Geometry check sheet. Reference: the model listing, model coordinates, mm. A direction names the side the tool comes from. Give positions to 0.01 mm unless a question says otherwise; leave off trailing zeros. Order: outer loops, then holes, each group sorted by start corner. A loop starts at its lowest first (then second) coordinate and runs counter-clockwise, first axis right, second up.
from build123d import *

# Parameters (mm, degrees)
SKETCH1_W           = 146.05
SKETCH1_H           = 146.05
SKETCH1_R           = 3.175
BOSS_EXTRUDE1_DEPTH = 3.175
SKETCH4_W           = 12.7
SKETCH4_H           = 12.7
BOSS_EXTRUDE4_DEPTH = 9.525
SKETCH6_W           = 5.935
SKETCH6_H           = 6
CUT_EXTRUDE2_DEPTH  = 150
SKETCH7_W           = 5.935
SKETCH7_H           = 6
CUT_EXTRUDE3_DEPTH  = 15
SKETCH2_R           = 1.5
CUT_EXTRUDE4_DEPTH  = 15
FILLET2_R           = 3.175


with BuildPart() as part:
    # Sketch1 → Boss-Extrude1 (new body)
    with BuildSketch(Plane(origin=(0, 0, 0), x_dir=(1, 0, 0), z_dir=(0, 1, 0))):
        with Locations((73.025, 73.025)):
            Rectangle(SKETCH1_W, SKETCH1_H)
        with Locations(Location((133.35, 12.7, 0), (0, 0, 270))):
            Circle(SKETCH1_R, mode=Mode.SUBTRACT)
        with Locations(Location((82.55, 12.7, 0), (0, 0, 270))):
            Circle(SKETCH1_R, mode=Mode.SUBTRACT)
    extrude(amount=BOSS_EXTRUDE1_DEPTH)

    # Sketch4 → Boss-Extrude4 (add)
    with BuildSketch(Plane(origin=(0, 3.175, 0), x_dir=(1, 0, 0), z_dir=(0, 1, 0))):
        with Locations((10.648879027, 12.7)):
            Rectangle(SKETCH4_W, SKETCH4_H)
        with Locations((10.648879027, 125.73)):
            Rectangle(SKETCH4_W, SKETCH4_H)
        with Locations((133.838879027, 125.73)):
            Rectangle(SKETCH4_W, SKETCH4_H)
    extrude(amount=BOSS_EXTRUDE4_DEPTH)

    # Sketch6 → Cut-Extrude2 (cut)
    with BuildSketch(Plane.XY.offset(-6.35)):
        with Locations((10.648879027, 6.175)):
            Rectangle(SKETCH6_W, SKETCH6_H)
    extrude(amount=-CUT_EXTRUDE2_DEPTH, mode=Mode.SUBTRACT)

    # Sketch7 → Cut-Extrude3 (cut)
    with BuildSketch(Plane.XY.offset(-119.38)):
        with Locations((133.838879027, 6.175)):
            Rectangle(SKETCH7_W, SKETCH7_H)
    extrude(amount=-CUT_EXTRUDE3_DEPTH, mode=Mode.SUBTRACT)

    # Sketch2 → Cut-Extrude4 (cut)
    with BuildSketch(Plane(origin=(0, 3.175, 0), x_dir=(1, 0, 0), z_dir=(0, 1, 0))):
        with Locations(Location((10.648879027, 125.73, 0), (0, 0, 90))):
            Circle(SKETCH2_R)
        with Locations(Location((133.838879027, 125.73, 0), (0, 0, 180))):
            Circle(SKETCH2_R)
        with Locations(Location((10.648879027, 12.7, 0), (0, 0, 90))):
            Circle(SKETCH2_R)
    extrude(amount=CUT_EXTRUDE4_DEPTH, mode=Mode.SUBTRACT)

    # Fillet2
    # the kernel refuses this fillet: 3.175 mm, written as the material it adds along each edge
    with BuildSketch(Plane(origin=(136.806379027, 9.175, -119.38), x_dir=(0, -1, 0), z_dir=(0, 0, -1))) as fillet2_piece_1_section:
        with BuildLine():
            CenterArc((FILLET2_R, FILLET2_R), FILLET2_R, 180, 90)
            Line((0, FILLET2_R), (0, 0))
            Line((0, 0), (FILLET2_R, 0))
        make_face()
    fillet2_piece_1 = extrude(amount=12.7, mode=Mode.PRIVATE)
    fillet2_piece_1 = fillet2_piece_1 - Plane(origin=(133.838879027, 8.440537645, -125.73), x_dir=(-1, 0, 0), z_dir=(0, -1, 0)) * Cylinder(1.5, 39, mode=Mode.PRIVATE)
    add(fillet2_piece_1)
    with BuildSketch(Plane(origin=(130.871379027, 9.175, -119.38), x_dir=(0, -1, 0), z_dir=(0, 0, -1))) as fillet2_piece_2_section:
        with BuildLine():
            CenterArc((FILLET2_R, -FILLET2_R), FILLET2_R, 90, 90)
            Line((0, -FILLET2_R), (0, 0))
            Line((0, 0), (FILLET2_R, 0))
        make_face()
    fillet2_piece_2 = extrude(amount=12.7, mode=Mode.PRIVATE)
    fillet2_piece_2 = fillet2_piece_2 - Plane(origin=(133.838879027, 8.44053751, -125.73), x_dir=(-1, 0, 0), z_dir=(0, -1, 0)) * Cylinder(1.5, 39, mode=Mode.PRIVATE)
    add(fillet2_piece_2)
    with BuildSketch(Plane(origin=(13.616379027, 9.175, -119.38), x_dir=(0, -1, 0), z_dir=(0, 0, -1))) as fillet2_piece_3_section:
        with BuildLine():
            CenterArc((FILLET2_R, FILLET2_R), FILLET2_R, 180, 90)
            Line((0, FILLET2_R), (0, 0))
            Line((0, 0), (FILLET2_R, 0))
        make_face()
    fillet2_piece_3 = extrude(amount=12.7, mode=Mode.PRIVATE)
    fillet2_piece_3 = fillet2_piece_3 - Plane(origin=(10.648879027, 8.440537543, -125.73), x_dir=(0, 0, -1), z_dir=(0, -1, 0)) * Cylinder(1.5, 39, mode=Mode.PRIVATE)
    add(fillet2_piece_3)
    with BuildSketch(Plane(origin=(7.681379027, 9.175, -119.38), x_dir=(0, -1, 0), z_dir=(0, 0, -1))) as fillet2_piece_4_section:
        with BuildLine():
            CenterArc((FILLET2_R, -FILLET2_R), FILLET2_R, 90, 90)
            Line((0, -FILLET2_R), (0, 0))
            Line((0, 0), (FILLET2_R, 0))
        make_face()
    fillet2_piece_4 = extrude(amount=12.7, mode=Mode.PRIVATE)
    fillet2_piece_4 = fillet2_piece_4 - Plane(origin=(10.648879027, 8.440537622, -125.73), x_dir=(0, 0, -1), z_dir=(0, -1, 0)) * Cylinder(1.5, 39, mode=Mode.PRIVATE)
    add(fillet2_piece_4)
    with BuildSketch(Plane(origin=(13.616379027, 9.175, -6.35), x_dir=(0, -1, 0), z_dir=(0, 0, -1))) as fillet2_piece_5_section:
        with BuildLine():
            CenterArc((FILLET2_R, FILLET2_R), FILLET2_R, 180, 90)
            Line((0, FILLET2_R), (0, 0))
            Line((0, 0), (FILLET2_R, 0))
        make_face()
    fillet2_piece_5 = extrude(amount=12.7, mode=Mode.PRIVATE)
    fillet2_piece_5 = fillet2_piece_5 - Plane(origin=(10.648879027, 8.440537543, -12.7), x_dir=(0, 0, -1), z_dir=(0, -1, 0)) * Cylinder(1.5, 39, mode=Mode.PRIVATE)
    add(fillet2_piece_5)
    with BuildSketch(Plane(origin=(7.681379027, 9.175, -6.35), x_dir=(0, -1, 0), z_dir=(0, 0, -1))) as fillet2_piece_6_section:
        with BuildLine():
            CenterArc((FILLET2_R, -FILLET2_R), FILLET2_R, 90, 90)
            Line((0, -FILLET2_R), (0, 0))
            Line((0, 0), (FILLET2_R, 0))
        make_face()
    fillet2_piece_6 = extrude(amount=12.7, mode=Mode.PRIVATE)
    fillet2_piece_6 = fillet2_piece_6 - Plane(origin=(10.648879027, 8.440537622, -12.7), x_dir=(0, 0, -1), z_dir=(0, -1, 0)) * Cylinder(1.5, 39, mode=Mode.PRIVATE)
    add(fillet2_piece_6)


solid = part.part
Item 1: Sectioned sample at B-B (z = -98). Enter the section's corners in (x, y) (3 decimals).
Reported:
outline: (0, 0) - (146.05, 0) - (146.05, 3.175) - (0, 3.175) - close
Item 2: Gauge pin test, flat ends, axial feed: pin 1 (3 mm diameter, centred on y = 4.5, z = -11.5, fed in from -X); pin 2 (0.8 mm diameter, centred on y = 4, z = -126, fed in from +X); pin 3 (3 mm diameter, centred on y = 6.5, z = -128, fed in from -X); pin 4 (3 mm diameter, centred on y = 6, z = -48.5, fed in from -X). Record the tip position at first contact, or that the pin passes through.
Reported:
pin 1: stops at x = 0
pin 2: stops at x = 140.19
pin 3: stops at x = 4.3
pin 4: passes through
Item 3: Draft check along X on faces 6 (the flat face through (4.299, 8, -13)), 7 (the cylindrical face through (8.52, 8.15, -125.64)), 8 (the flat face through (140.189, 8, -126)), 9 (the flat face through (72, 2, 0)). Enter one of: released by +X, released by -X, zero draft, split by the parting line, or undercut.
Reported:
face 6: released by -X
face 7: undercut
face 8: released by +X
face 9: zero draft
Item 4: Scan lines: L1, parallel to X at y = 11.3, z = -125.73; L2, parallel to X at y = 1.2, z = -12.7 (3 decimals); L3, parallel to Z at x = 135.5, y = 11.25. Record each from-to range of solid material in increasing order.
Reported:
L1: x = 4.3 to 9.15, 12.15 to 17, 127.49 to 132.34, 135.34 to 140.19
L2: x = 0 to 79.375, 85.725 to 130.175, 136.525 to 146.05
L3: z = -132.08 to -119.38
Item 5: Sectioned sample at A-A (x = 82.55). Enter the section's corners in (y, z) (3 decimals), and give its area (3 significant figures).
Reported:
outline: (0, -146.05) - (3.175, -146.05) - (3.175, -15.875) - (0, -15.875) - close; (0, -9.525) - (3.175, -9.525) - (3.175, 0) - (0, 0) - close
area: 444 mm2
Item 6: Set-up check for faces 1 (the cylindrical face through (135.93, 8.19, -125.64)), 2 (the flat face through (11, 10, -19.05)), 3 (the flat face through (11, 10, -6.35)), 4 (the flat face through (16.999, 8, -13)), 5 (the flat face through (134, 10, -132.08)): record each of +Z, -Z, +X, -X, +Y, -Y from which the full face is reachable in a straight line by a thin tool's end or side.
Reported:
face 1: +Z, -Z
face 2: +X, -X, +Y
face 3: +Z, +X, -X, +Y
face 4: +Z, -Z, +X, +Y
face 5: -Z, +X, -X, +Y
